Geometry: final body of the model. Coordinates: model frame, mm. Face numbers are marked on the shaded views. A direction names the side the tool comes from. Coordinates: 2 decimals unless noted, no trailing zeros. Write each loop counter-clockwise with the first axis right and the second up, starting at its lowest first coordinate (ties: lowest second). Pieces come first, ordered by that corner, then holes. Notation, with made-up numbers: (37.25, 32.5) -> (43.25, 32.5) arc R21 cw to (43.25, 41.5) -> close; hole circle Ø1 at (-14.75, 28). An arc over 180 degrees is marked (long way). One line per item, written item: value.
```python
from build123d import *

# Parameters (mm, degrees)
SKETCH1_W               = 76
SKETCH1_H               = 29
BOSS_EXTRUDE1_DEPTH     = 4
SKETCH2_W               = 4
SKETCH2_H               = 29
BOSS_EXTRUDE2_DEPTH     = 32
CUT_EXTRUDE1_REACH      = 87.336
CUT_EXTRUDE2_DEPTH      = 82.793948581
CUT_EXTRUDE2_DEPTH_BACK = 82.793948581
SKETCH4_R               = 1.843066456


with BuildPart() as part:
    # Sketch1 → Boss-Extrude1 (new body)
    with BuildSketch(Plane(origin=(0, 0, 0), x_dir=(1, 0, 0), z_dir=(0, 1, 0))):
        Rectangle(SKETCH1_W, SKETCH1_H)
    extrude(amount=BOSS_EXTRUDE1_DEPTH)

    # Sketch2 → Boss-Extrude2 (add)
    with BuildSketch(Plane(origin=(0, 4, 0), x_dir=(1, 0, 0), z_dir=(0, 1, 0))):
        with Locations((-36, 0)):
            Rectangle(SKETCH2_W, SKETCH2_H)
        with Locations((36, 0)):
            Rectangle(SKETCH2_W, SKETCH2_H)
    extrude(amount=BOSS_EXTRUDE2_DEPTH)

    # Cut-Extrude1: up to this face of the body (flat: up to its plane)
    cut_extrude1_end = Plane(part.part.faces().sort_by_distance((38, 18, 0))[0])
    # Sketch3 → Cut-Extrude1 (cut, up to the picked face)
    with BuildSketch(Plane.ZY.offset(38), mode=Mode.PRIVATE) as cut_extrude1_sk1:
        with BuildLine():
            Line((14.5, 4), (14.5, 36))
            Line((14.5, 36), (4, 36))
            add(Edge.make_bspline(
                [(14.5, 4), (13.053007325, 36), (4, 36)],
                knots=[0, 0, 0, 1, 1, 1], degree=2))
        make_face()
    cut_extrude1_tool1 = split(extrude(cut_extrude1_sk1.sketch, amount=-CUT_EXTRUDE1_REACH, mode=Mode.PRIVATE), bisect_by=cut_extrude1_end, keep=Keep.BOTH, mode=Mode.PRIVATE)
    # Sketch3 → Cut-Extrude1 (cut, up to the picked face)
    with BuildSketch(Plane.ZY.offset(38), mode=Mode.PRIVATE) as cut_extrude1_sk2:
        with BuildLine():
            Line((-4, 36), (-14.5, 36))
            Line((-14.5, 36), (-14.5, 4))
            add(Edge.make_bspline(
                [(-14.5, 4), (-13.053007325, 36), (-4, 36)],
                knots=[0, 0, 0, 1, 1, 1], degree=2))
        make_face()
    cut_extrude1_tool2 = split(extrude(cut_extrude1_sk2.sketch, amount=-CUT_EXTRUDE1_REACH, mode=Mode.PRIVATE), bisect_by=cut_extrude1_end, keep=Keep.BOTH, mode=Mode.PRIVATE)
    add(cut_extrude1_tool1.solids().sort_by(Axis((-38, 28.217177, 12.337471), (1, 0, 0)))[0], mode=Mode.SUBTRACT)
    add(cut_extrude1_tool2.solids().sort_by(Axis((-38, 28.217177, -12.337471), (1, 0, 0)))[0], mode=Mode.SUBTRACT)

    # Sketch4 → Cut-Extrude2 (cut, two sides: drawn at the far end of the back side and taken through both)
    with BuildSketch(Plane.ZY.offset(-34).offset(-CUT_EXTRUDE2_DEPTH_BACK)):
        with Locations((0, 28)):
            Circle(SKETCH4_R)
    extrude(amount=CUT_EXTRUDE2_DEPTH + CUT_EXTRUDE2_DEPTH_BACK, mode=Mode.SUBTRACT)


solid = part.part
```
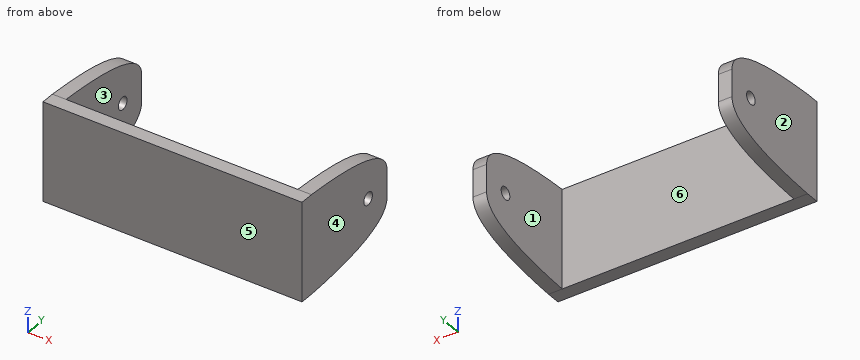
(1) Section B-B (y = 28). State how many separate pieces and enclosed holes the cut face has, then the cut area to 3 significant figures.
Responses:
separate pieces: 4
enclosed holes: 0
area: 149 mm2
(2) Line query: line 1 (X direction, y = 21.5, z = -4.75); line 2 (Y direction, x = -36.1, z = 0); line 3 (Y direction, x = 12, z = 8.25). Output: solid intervals per line, ascending. Write a range as [from, to].
Responses:
line 1: x = [-38, -34], [34, 38]
line 2: y = [0, 26.16], [29.84, 36]
line 3: y = [0, 4]
(3) Section A-A (z = 0). Return the cut outline in (x, y).
Responses:
outline: (-38, 0) -> (38, 0) -> (38, 26.16) -> (34, 26.16) -> (34, 4) -> (-34, 4) -> (-34, 26.16) -> (-38, 26.16) -> close; (-38, 29.84) -> (-34, 29.84) -> (-34, 36) -> (-38, 36) -> close; (34, 29.84) -> (38, 29.84) -> (38, 36) -> (34, 36) -> close
(4) Section C-C (x = 15.5). Return the cut outline in (y, z), then the cut area to 3 significant figures.
Responses:
outline: (0, -14.5) -> (4, -14.5) -> (4, 14.5) -> (0, 14.5) -> close
area: 116 mm2
(5) First-contact query: pin 1 (2 mm diameter, centred on x = -27, z = 8, fed in from +Y). Flat tip, straight axial feed; report the tip coordinate or a pass-through.
Responses:
pin 1: stops at y = 4
(6) Reachability of the marked faces 5 and 6 from +Z, -Z, +X, -X, +Y, -Y: full face, straight path, thin tool, end or side. Return the list, or none.
Responses:
face 5: +Z, -Z, +X, -X, -Y
face 6: +Z, -Z, +Y
(7) Pull-direction query (X, two-part tool) for the marked faces 1, 2, 3 and 4; classes: released by +X, released by -X, zero draft, split by the parting line, or undercut.
Responses:
face 1: undercut
face 2: released by -X
face 3: undercut
face 4: released by +X
